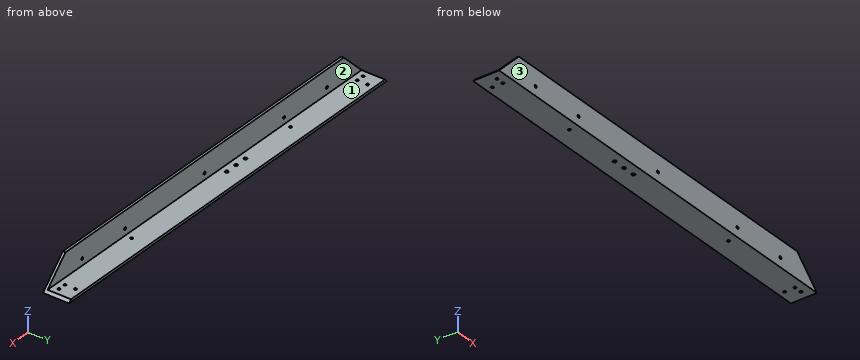
from build123d import *

# Parameters (mm, degrees)
BOSS_EXTRUDE1_DEPTH          = 510
CHAMFER6_SIZE                = 31.75
CHAMFER7_SIZE                = 31.75
TOPHOLES_SKETCH3_R           = 1.5875
TOPHOLES_CUT_EXTRUDE2_DEPTH  = 512.785690622
BACKHOLES_SKETCH4_R          = 1.5875
BACKHOLES_SKETCH4_R_2        = 2
BACKHOLES_CUT_EXTRUDE3_DEPTH = 512.785690622


with BuildPart() as part:
    # Sketch1 → Boss-Extrude1 (new body)
    with BuildSketch(Plane(origin=(0, 0, 0), x_dir=(0, 0, -1), z_dir=(1, 0, 0))):
        Polygon((0, 0), (-31.75, 0), (-31.75, 3.175), (-3.175, 3.175), (-3.175, 31.75), (0, 31.75), align=None)
    extrude(amount=BOSS_EXTRUDE1_DEPTH)

    # Chamfer6
    chamfer6_edges = [part.edges().sort_by_distance(p)[0] for p in [
        (510, 1.5875, 31.75),
    ]]
    chamfer(chamfer6_edges, length=CHAMFER6_SIZE - 0.0001)  # a hair under: the kernel refuses the full size

    # Chamfer7
    chamfer7_edges = [part.edges().sort_by_distance(p)[0] for p in [
        (0, 1.5875, 31.75),
    ]]
    chamfer(chamfer7_edges, length=CHAMFER7_SIZE - 0.0001)  # a hair under: the kernel refuses the full size

    # TopHoles-Sketch3 → TopHoles-Cut-Extrude2 (cut, through all)
    with BuildSketch(Plane(origin=(0, 3.175, 0), x_dir=(1, 0, 0), z_dir=(0, 1, 0))):
        with Locations(Location((451.2625, -11.1125, 0), (0, 0, 270))):
            Circle(TOPHOLES_SKETCH3_R)
        with Locations(Location((58.7375, -11.1125, 0), (0, 0, 270))):
            Circle(TOPHOLES_SKETCH3_R)
        with Locations(Location((127.5, -11.1125, 0), (0, 0, 270))):
            Circle(TOPHOLES_SKETCH3_R)
        with Locations(Location((255, -11.1125, 0), (0, 0, 270))):
            Circle(TOPHOLES_SKETCH3_R)
        with Locations(Location((382.5, -11.1125, 0), (0, 0, 270))):
            Circle(TOPHOLES_SKETCH3_R)
    extrude(amount=-TOPHOLES_CUT_EXTRUDE2_DEPTH, mode=Mode.SUBTRACT)

    # BackHoles-Sketch4 → BackHoles-Cut-Extrude3 (cut, through all)
    with BuildSketch(Plane.XY.offset(3.175)):
        with Locations((489.3625, 23.8125)):
            Circle(BACKHOLES_SKETCH4_R)
        with Locations((20.6375, 23.8125)):
            Circle(BACKHOLES_SKETCH4_R)
        with Locations((11.1125, 11.1125)):
            Circle(BACKHOLES_SKETCH4_R)
        with Locations((20.6375, 11.1125)):
            Circle(BACKHOLES_SKETCH4_R)
        with Locations((489.3625, 11.1125)):
            Circle(BACKHOLES_SKETCH4_R)
        with Locations((498.8875, 11.1125)):
            Circle(BACKHOLES_SKETCH4_R)
        with Locations((200, 11.1125)):
            Circle(BACKHOLES_SKETCH4_R_2)
        with Locations((215, 11.1125)):
            Circle(BACKHOLES_SKETCH4_R_2)
        with Locations((230, 11.1125)):
            Circle(BACKHOLES_SKETCH4_R_2)
        with Locations((127.5, 11.1125)):
            Circle(BACKHOLES_SKETCH4_R)
        with Locations((382.5, 11.1125)):
            Circle(BACKHOLES_SKETCH4_R)
    extrude(amount=-BACKHOLES_CUT_EXTRUDE3_DEPTH, mode=Mode.SUBTRACT)


solid = part.part
Read the model definition and answer for the solid it produces. Units are mm, in the model's axes. Face numbers are marked on the shaded views. Coordinates: 2 decimals unless noted, no trailing zeros. Write each loop counter-clockwise with the first axis right and the second up, starting at its lowest first coordinate (ties: lowest second). Pieces come first, ordered by that corner, then holes. Notation, with made-up numbers: (17, 10) - (32, 10) arc R18 cw to (32, 43) - close; hole circle Ø9 at (67.5, -14.75). An arc over 180 degrees is marked (long way). One line per question, with ' | ' between items.
Q1. Find section A-A, the plane x = 42. Write down the section's boundary in (y, z) (3 decimals), plus the area to 3 significant figures.
Result set:
outline: (0, 0) - (31.75, 0) - (31.75, 3.175) - (3.175, 3.175) - (3.175, 31.75) - (0, 31.75) - close | area: 192 mm^2
Q2. Find section B-B, the plane z = 18.5. Write down the section's boundary in (x, y) (3 decimals), plus the area to 3 significant figures.
Result set:
outline: (18.5, 0) - (491.5, 0) - (491.5, 3.175) - (18.5, 3.175) - close | area: 1,500 mm^2
Q3. Consider L1, parallel to Y at x = 215, z = 2.2; L2, parallel to Y at x = 383, z = 3; L3, parallel to Z at x = 382.5, y = 1.3 (3 decimals). Determine where each line is inside the solid, lowest interval first. Write a range as [from, to].
Result set:
L1: [0, 9.11], [13.11, 31.75] | L2: [0, 9.61], [12.62, 31.75] | L3: [0, 9.525], [12.7, 31.75]
Q4. Each of these flat-tipped pins is pushed along its axis until it touches: P1, Ø4, axis at x = 11.11, y = 11.11, coming from the +Z side (3 decimals); P2, Ø10, axis at y = 20.5, z = 7.5, coming from the -X side; P3, Ø6, axis at x = 150.5, z = 8, coming from the +Y side (3 decimals). Where does it stop, or does it pass through?
Result set:
P1: z = 3.175 | P2: x = 2.5 | P3: y = 3.175
Q5. Determine the mould class of the marked faces 1, 2 and 3 for opening direction Y: +Y half, -Y half, draft (parallel to the pull), parting line (faces both ways), or undercut.
Result set:
face 1: draft | face 2: +Y half | face 3: -Y half
